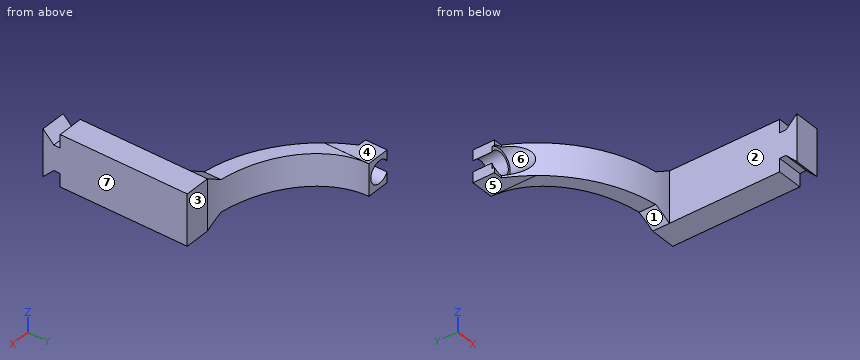
Autodesk Inventor part; units mm, degrees
ref_plane "YZ Plane" through (0, 0, 0) normal (1, 0, 0) x (0, 1, 0)
ref_plane "XZ Plane" through (0, 0, 0) normal (0, 1, 0) x (-1, 0, 0)
ref_plane "XY Plane" through (0, 0, 0) normal (0, 0, 1) x (1, 0, 0)
sketch "Sketch1" plane through (0, 0, 0) normal (1, 0, 0) x (0, 1, 0)
  line L0 (0, 0) -> (0, 3.9)
  line L1 (0, 0) -> (0, -3.9)
  line L2 (0, 3.9) -> (-3.3941, 7.2941)
  line L3 (0, 3.9) -> (4.8, 3.9) construction
  line L4 (0, -3.9) -> (-3.3941, -7.2941)
  line L5 (0, -3.9) -> (4.8, -3.9) construction
  line L6 (-3.3941, -7.2941) -> (-3.3941, 7.2941)
  dimension "d0" = 3.9
  dimension "d1" = 3.9
  dimension "d2" = 4.8
  dimension "d3" = 135
  dimension "d4" = 4.8
  dimension "d5" = 135
extrude "Extrusion1" add sketch "Sketch1" along normal blind 8
sketch "Sketch2" plane through (0, 0, 3.9) normal (0, 1, 0) x (1, 0, 0)
  line L0 (0, -3.3941) -> (0, 11.1941)
  line L1 (0, -0.0082) -> (8, -0.0082)
  line L2 (8, -0.0082) -> (8, 7.7918)
  line L3 (8, 7.7918) -> (0, 7.7918)
  line L4 (0, 7.7918) -> (0, -0.0082)
  point P0 (0, 3.9)
  dimension "d8" = 8
  dimension "d9" = 7.8
extrude "Extrusion2" add sketch "Sketch2" along normal blind 2
sketch "Sketch3" plane through (0, 2, 3.9) normal (0, 1, 0) x (1, 0, 0)
  line L0 (8, -4.1082) -> (0, -4.1082)
  line L1 (0, -4.1082) -> (0, 11.8918)
  line L2 (0, 11.8918) -> (8, 11.8918)
  line L3 (8, 11.8918) -> (8, -4.1082)
  line L4 (8, -4.1082) -> (0, 11.8918) construction
  line L5 (0, -4.1082) -> (8, 11.8918) construction
  line L6 (8, 7.7918) -> (0, 7.7918)
  point P0 (0, 3.9)
  point P1 (4, 3.8918)
  dimension "d12" = 8
  dimension "d13" = 16
  dimension "d14" = 3.9
  dimension "d15" = 4
extrude "Extrusion3" add sketch "Sketch3" along normal blind 64.606
sketch "Sketch4" plane through (0, 0, 0) normal (-1, 0, 0) x (0, 0, 1)
  line L0 (-7.9918, 2) -> (-7.9918, 66.606)
  line L1 (8.0082, 2) -> (8.0082, 66.606)
  line L2 (-7.9918, 66.606) -> (8.0082, 66.606)
  line L3 (8.0082, 66.606) -> (8.0082, 36.606)
  line L4 (8.0082, 36.606) -> (-7.9918, 36.606)
  line L5 (-7.9918, 36.606) -> (-7.9918, 66.606)
  point P0 (0, 0)
  point P1 (8.0082, 66.606)
  point P2 (-7.9918, 36.606)
  dimension "d18" = 30
extrude "Extrusion4" add sketch "Sketch4" along normal blind 40
sketch "Sketch5" plane through (0, 66.606, 3.9) normal (0, 1, 0) x (1, 0, 0)
  circle A0 centre (-37, 3.8918) radius 3.45
  line L0 (-40, -4.1082) -> (-40, 11.8918)
  line L1 (8, 11.8918) -> (-40, 11.8918)
  point P0 (0, 3.9)
  point P1 (-40, 5.5955)
  point P2 (-40, 2.1882)
  dimension "d21" = 6.9
  dimension "d22" = 3
  dimension "d53" = 8
sketch "Sketch6" plane through (0, 2, 8.0082) normal (0, 0, 1) x (1, 0, 0)
  point P0 (0, -2)
sketch "Sketch7" plane through (0, 2, 8.0082) normal (0, 0, 1) x (1, 0, 0)
  point P0 (0, -2)
sketch "Sketch10" plane through (0, 2, 8.0082) normal (0, 0, 1) x (1, 0, 0)
  ellipse E0 centre (0, 64.6805) end of major axis (0, 39.8349) minor radius 32.7521
  line L0 (8, 64.606) -> (-40, 64.606)
  line L1 (0, 39.8349) -> (8, 39.8349)
  line L2 (8, 39.8349) -> (8, 64.606)
  line L3 (8, 64.606) -> (0, 64.606)
  line L4 (0, 64.606) -> (0, 39.8349)
  point P0 (0, -2)
  point P1 (8, 40.5875)
extrude "Extrusion8" cut sketch "Sketch10" against normal through all
sketch "Sketch13" plane through (0, 36.606, -7.9918) normal (0, -1, 0) x (1, 0, 0)
  circle A0 centre (-37.1694, 8) radius 4.375
  line L0 (0, 16) -> (-40, 16)
  point P0 (0, 7.9918)
  dimension "d37" = 8.75
  dimension "d46" = 8
extrude "Extrusion9" cut sketch "Sketch13" against normal blind 24
extrude "Extrusion10" cut sketch "Sketch5" against normal blind 24
sketch "Sketch14" plane through (8, 2, -7.9918) normal (0, 0, -1) x (-1, 0, 0)
  line L0 (48, 34.606) -> (40.7944, 34.606)
  line L1 (45.2609, 34.606) -> (48, 34.606)
  line L2 (48, 34.606) -> (48, 57.8825)
  line L3 (48, 57.8825) -> (45.2609, 57.8825)
  line L4 (45.2609, 57.8825) -> (45.2609, 34.606)
  point P0 (8, -2)
extrude "Extrusion11" cut sketch "Sketch14" against normal blind 24
sketch "Sketch15" plane through (0, 2, 8.0082) normal (0, 0, 1) x (1, 0, 0)
  line L0 (-37.2609, 57.8825) -> (-37.2609, 34.606)
  line L1 (0, 34.606) -> (-37.2609, 34.606)
  arc A0 (-37.2609, 57.8825) -> (0, 34.606) centre (-0.1523, 75.824) ccw
  point P0 (0, -2)
  point P1 (-0.3046, 34.606)
extrude "Extrusion12" cut sketch "Sketch15" against normal through all
sketch "Sketch16" plane through (0, 66.606, 3.9) normal (0, 1, 0) x (1, 0, 0)
  line L0 (-40, 5.5955) -> (-40, 11.8918)
  line L1 (-32.752, 11.8918) -> (-40, 11.8918)
  line L2 (-32.752, -4.1082) -> (-32.752, 11.8918)
  line L3 (-40, 11.8918) -> (-32.752, 11.8918)
  line L4 (-32.752, 11.8918) -> (-32.752, 8.8918)
  line L5 (-32.752, 8.8918) -> (-40, 8.8918)
  line L6 (-40, 8.8918) -> (-40, 11.8918)
  line L7 (0, 11.8918) -> (0, 7.7918)
  line L8 (0, 11.8918) -> (-5, 11.8918)
  line L9 (-5, 11.8918) -> (-5, 8.8755)
  line L10 (-5, 8.8755) -> (0, 8.8755)
  line L11 (0, 8.8755) -> (0, 11.8918)
  line L12 (-5, 8.8755) -> (-32.752, 8.8755)
  line L13 (-32.752, 8.8755) -> (-32.752, 11.8918)
  line L14 (-32.752, 11.8918) -> (-5, 11.8918)
  line L15 (-5, 11.8918) -> (-5, 8.8755)
  line L16 (0, 11.8918) -> (-5, 8.8755)
  line L17 (0, 3.8918) -> (-40, 3.8918)
  line L18 (-40, 2.1882) -> (-40, -4.1082)
  line L19 (-32.752, -4.1082) -> (-40, -4.1082)
  line L20 (-32.752, 11.8918) -> (-32.752, -4.1082)
  line L21 (-40, -4.1082) -> (-32.752, -4.1082)
  line L22 (-32.752, -4.1082) -> (-32.752, -1.1082)
  line L23 (-32.752, -1.1082) -> (-40, -1.1082)
  line L24 (-40, -1.1082) -> (-40, -4.1082)
  line L25 (0, -4.1082) -> (0, -0.0082)
  line L26 (0, -4.1082) -> (-5, -4.1082)
  line L27 (-5, -4.1082) -> (-5, -1.0918)
  line L28 (-5, -1.0918) -> (0, -1.0918)
  line L29 (0, -1.0918) -> (0, -4.1082)
  line L30 (-5, -1.0918) -> (-32.752, -1.0918)
  line L31 (-32.752, -1.0918) -> (-32.752, -4.1082)
  line L32 (-32.752, -4.1082) -> (-5, -4.1082)
  line L33 (-5, -4.1082) -> (-5, -1.0918)
  line L34 (0, -4.1082) -> (-5, -1.0918)
  point P0 (0, -1.0918)
  dimension "d48" = 3
  dimension "d49" = 5
  dimension "d52" = 8
extrude "Extrusion13" cut sketch "Sketch16" against normal through all contours L30 L27 L32 L2 | L0 L1 L2 L5 | L2 L14 L9 L12 | L8 L16 L9 | L2 L19 L18 L23 | L34 L26 L27
properties part number "Pasteur_holder_V2"
Here's how the part is built. I have some questions about the finished solid (model axes, mm). Face numbers are marked on the shaded views. A direction names the side the tool comes from. Give positions to 0.01 mm unless a question says otherwise; leave off trailing zeros. Order: outer loops, then holes, each group sorted by start corner. A loop starts at its lowest first (then second) coordinate and runs counter-clockwise, first axis right, second up. Notation, with made-up numbers: M 78.5,26 L 132.5,26 A19 cw 132.5,55 Z; hole C -18,27.5 d7. An arc over 180 degrees is marked long. Use a Markdown table: item, result. Add a question column.
1. On a 3-axis mill with a long thin cutter (end or side, diameter ignored), from which of +Z, -Z, +X, -X, +Y, -Y can I reach the whole of each face in a straight line? I mean the marked faces 1, 2 and 3. Say none if no direction works.
2. If we mould it in two halves opening along Z, with no side actions, what happens to the marked faces 4, 5, 6 and 7? For each: +Z half, -Z half, draft (parallel to the pull), parting line (faces both ways), or undercut.
3. I need wall thicknesses on probe 1 along Z at (x, y) = (-37, 64.8); probe 2 along X at (y, z) = (31, -5.5); probe 3 along X at (y, z) = (63, 2.5). Which ranges of each line are inside material? Lowest first, please. Write a range as from..to.
4. Suppose I cut it at A-A (y = 41). List the corners of the cut face in (x, z) for me.
5. For pin 1 Ø0.5 at (x, z) = (-38.5, 4) entering from -Y; pin 2 Ø4 at (y, z) = (55, -0.5) entering from +X; pin 3 Ø6 at (x, y) = (-34.5, 57) entering from -Z; pin 4 Ø3 at (x, y) = (-3, 4) entering from +Z, each with a flat end and sliding along its axis, tell me the tip position at first contact or that it passes through.
Results list:
| question | item | result |
|---|---|---|
| 1 | face 1 | -Z, -X, +Y, -Y |
| 1 | face 2 | +Z, -Z, -X, -Y |
| 1 | face 3 | +Z, -Z, +X, +Y |
| 2 | face 4 | +Z half |
| 2 | face 5 | -Z half |
| 2 | face 6 | undercut |
| 2 | face 7 | draft |
| 3 | probe 1 | z = -4.99..-3.44, 3.46..5.01 |
| 3 | probe 2 | x = 0..8 |
| 3 | probe 3 | x = -40..-39.39, -34.61..-32.39 |
| 4 | outline | M -18.67,-4.98 L -5,-4.98 L 0,-7.99 L 8,-7.99 L 8,8.01 L 0,8.01 L -5,4.99 L -18.67,4.99 Z |
| 5 | pin 1 | stops at y = 59.88 |
| 5 | pin 2 | stops at x = -27.34 |
| 5 | pin 3 | stops at z = -4.99 |
| 5 | pin 4 | passes through |
